from build123d import *

# Parameters (mm, degrees)
SKETCH_1_R               = 8
EXTRUDE_1_DEPTH          = 700
SKETCH_2_R               = 4
CUT_EXTRUDE_1_DEPTH      = 9
CUT_EXTRUDE_1_DEPTH_BACK = 9
SKETCH_3_OUTSIDE_W       = 158.074
SKETCH_3_OUTSIDE_H       = 158.074
SKETCH_3_OUTSIDE_W_2     = 8
SKETCH_3_OUTSIDE_H_2     = 20
CUT_EXTRUDE_2_DEPTH      = 20
SKETCH_4_R               = 2.5
CUT_EXTRUDE_3_DEPTH      = 10


with BuildPart() as part:
    # 草图1 → 凸台-拉伸1 (new body)
    with BuildSketch(Plane(origin=(0, 0, 0), x_dir=(0, 0, -1), z_dir=(1, 0, 0))):
        Circle(SKETCH_1_R)
    extrude(amount=EXTRUDE_1_DEPTH)

    # 草图2 → 切除-拉伸1 (cut, two sides)
    with BuildSketch(Plane.XY) as cut_extrude_1_sk:
        with Locations((10, 0)):
            Circle(SKETCH_2_R)
    extrude(amount=CUT_EXTRUDE_1_DEPTH, mode=Mode.SUBTRACT)
    extrude(cut_extrude_1_sk.sketch, amount=-CUT_EXTRUDE_1_DEPTH_BACK, mode=Mode.SUBTRACT)

    # 草图3 outside → 切除-拉伸2 (cut)
    with BuildSketch(Plane.ZY):
        Rectangle(SKETCH_3_OUTSIDE_W, SKETCH_3_OUTSIDE_H)
        Rectangle(SKETCH_3_OUTSIDE_W_2, SKETCH_3_OUTSIDE_H_2, mode=Mode.SUBTRACT)
    extrude(amount=-CUT_EXTRUDE_2_DEPTH, mode=Mode.SUBTRACT)

    # 草图4 → 切除-拉伸3 (cut, symmetric)
    with BuildSketch(Plane(origin=(0, 0, 0), x_dir=(1, 0, 0), z_dir=(0, 1, 0))):
        with Locations((696, 0)):
            Circle(SKETCH_4_R)
    extrude(amount=CUT_EXTRUDE_3_DEPTH, both=True, mode=Mode.SUBTRACT)


solid = part.part
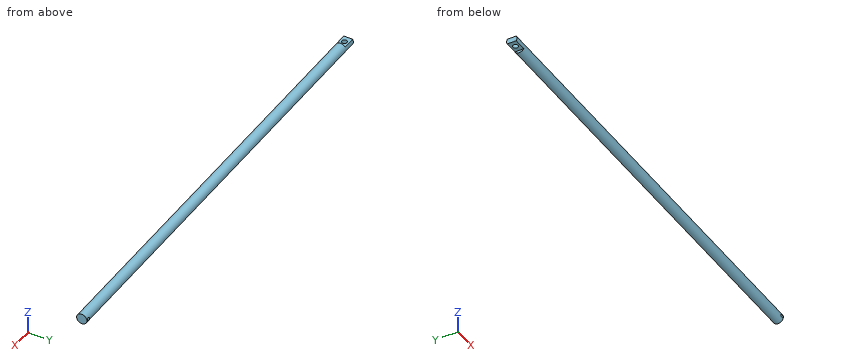
The model under review builds one solid part; all positions refer to its coordinate system, in mm. Give positions to 0.01 mm unless a question says otherwise; leave off trailing zeros. Order: outer loops, then holes, each group sorted by start corner. A loop starts at its lowest first (then second) coordinate and runs counter-clockwise, first axis right, second up. Notation, with made-up numbers: M -27.5,39 L 19.5,39 A17 ccw 19.5,72 Z; hole C 47.5,69 d6. An arc over 180 degrees is marked long. One line per question, with ' | ' between items. Start each with the question number.
1) Wall thickness on L1, parallel to X at y = -0.75, z = 0; L2, parallel to X at y = -0.25, z = 2.25; L3, parallel to Y at x = 10, z = 1: over which ranges is each line inside the solid? List them lowest first. Write a range as from..to.
2) Clearance check with flat-ended pins moving along their axes: P1, Ø1.2, axis at y = 2.5, z = 5, coming from the -X side; P2, Ø1, axis at x = 157.5, z = -3.5, coming from the +Y side; P3, Ø4, axis at x = 614.5, y = 4.5, coming from the -Z side. State where each tip first meets the part, or that it passes through.
3) Consider section B-B, the plane x = 145. Give the boundary of the cut face in (y, z), then the cut area to 3 significant figures.
4) Consider section A-A, the plane y = 0. Give the boundary of the cut face in (x, z), then the cut area to 3 significant figures.
Found:
1) L1: x = 0..6.07, 13.93..693.5, 698.5..700 | L2: x = 0..6.01, 13.99..694.91, 697.09..700 | L3: y = -7.94..-4, 4..7.94
2) P1: stops at x = 20 | P2: stops at y = 7.42 | P3: stops at z = -7.6
3) outline: C 0,0 d16 | area: 201 mm²
4) outline: M 0,-4 L 6,-4 L 6,4 L 0,4 Z; M 14,-4 L 20,-4 L 20,-8 L 700,-8 L 700,8 L 20,8 L 20,4 L 14,4 Z; hole C 696,0 d5 | area: 11,000 mm²
